For this review, take the finished solid that the model builds, in its own axes (mm). A direction names the side the tool comes from. Coordinates: 2 decimals unless noted, no trailing zeros. Loops run counter-clockwise (first coordinate to the right, second up) from the corner with the lowest first, then second, coordinate; pieces in that order, holes last. Notation, with made-up numbers: M 52.25,78.25 L 110.25,78.25 A23 ccw 110.25,95.25 Z; hole C 3,50.5 d3. An arc over 180 degrees is marked long. Put each result on its own line as item: value.
```python
from build123d import *


with BuildPart() as part:
    # Esquisse1 → Révolution1 (revolve)
    with BuildSketch(Plane.XY, mode=Mode.PRIVATE) as r_volution1_sk:
        Polygon((180, 0), (160, 0), (160, 47), (165, 47), (165, 12), (180, 12), align=None)
        Polygon((20, 0), (0, 0), (0, -20), (180, -20), (180, 0), (160, 0), align=None)
        Polygon((20, 0), (0, 0), (0, 12), (15, 12), (15, 47), (20, 47), align=None)
    revolve(r_volution1_sk.sketch.rotate(Axis((0, -30, 0), (1, 0, 0)), 90), axis=Axis((0, -30, 0), (1, 0, 0)))


solid = part.part
```
(1) Tool access review of faces 1 (the flat face through (180, -21, -9)), 2 (the flat face through (20, 3, -1)), 3 (the flat face through (165, 3, 33)): name each direction out of +Z, -Z, +X, -X, +Y, -Y from which nothing blocks a thin tool from reaching the whole face with its end or side.
Determined:
face 1: +Z, -Z, +X, +Y, -Y
face 2: none
face 3: +X
(2) Wall thickness on line 1 along X through (y, z) = (-81.5, 49); line 2 along Y through (x, z) = (139.5, 0); line 3 along Y through (x, z) = (42.5, 1): over which ranges is each line inside the solid? List them lowest first. Write a range as [from, to].
Determined:
line 1: x = [15, 20], [160, 165]
line 2: y = [-60, -40], [-20, 0]
line 3: y = [-59.98, -39.95], [-20.05, -0.02]
(3) Add section A-A (y = -30). Write out the cut boundary in (x, z), plus the area to 3 significant figures.
Determined:
outline: M 0,-42 L 15,-42 L 15,-77 L 20,-77 L 20,-30 L 160,-30 L 160,-77 L 165,-77 L 165,-42 L 180,-42 L 180,-10 L 0,-10 Z; M 0,10 L 180,10 L 180,42 L 165,42 L 165,77 L 160,77 L 160,30 L 20,30 L 20,77 L 15,77 L 15,42 L 0,42 Z
area: 8,860 mm^2
(4) Add section D-D (y = -52). Write out the cut boundary in (x, z).
Determined:
outline: M 0,-35.78 L 15,-35.78 L 15,-73.79 L 20,-73.79 L 20,-20.4 L 160,-20.4 L 160,-73.79 L 165,-73.79 L 165,-35.78 L 180,-35.78 L 180,35.78 L 165,35.78 L 165,73.79 L 160,73.79 L 160,20.4 L 20,20.4 L 20,73.79 L 15,73.79 L 15,35.78 L 0,35.78 Z
(5) Draft analysis for pull direction Y (two halves, no side actions). For faces 4 (the cylindrical face through (91.26, -20.24, -2.17)), 5 (the flat face through (15, 3, -33)), 6 (the cylindrical face through (7.605, 11.001, -9.105)), state which applies: +Y half, -Y half, draft (parallel to the pull), parting line (faces both ways), or undercut.
Determined:
face 4: undercut
face 5: draft
face 6: parting line
(6) Add section B-B (z = 51). Write out the cut boundary in (x, y).
Determined:
outline: M 15,-87.69 L 20,-87.69 L 20,27.69 L 15,27.69 Z; M 160,-87.69 L 165,-87.69 L 165,27.69 L 160,27.69 Z
(7) For pin 1 (3 mm diameter, centred on y = 18.5, z = -23.5, fed in from -X); pin 2 (2 mm diameter, centred on x = 57.5, y = -26, fed in from +Z); pin 3 (1 mm diameter, centred on y = 24.5, z = 36, fed in from +X); pin 4 (6 mm diameter, centred on y = -2, z = 9, fed in from -X), all flat-tipped, find the tip position at first contact; note any pin that passes through.
Determined:
pin 1: stops at x = 15
pin 2: stops at z = 29.85
pin 3: stops at x = 165
pin 4: stops at x = 0
(8) Add section C-C (x = 35.5). Write out the cut boundary in (y, z), plus the area to 3 significant figures.
Determined:
outline: C -30,0 d60; hole C -30,0 d20
area: 2,510 mm^2
